```python
from build123d import *

# Parameters (mm, degrees)
DODANIE_WYCI_GNI_CIE1_DEPTH      = 0.5
DODANIE_WYCI_GNI_CIE1_DEPTH_BACK = 2
DODANIE_WYCI_GNI_CIE2_DEPTH      = 5.5
DODANIE_WYCI_GNI_CIE3_DEPTH      = 1.5
ZAOKR_GLENIE1_R                  = 2
SZKIC6_W                         = 66.685530181
SZKIC6_H                         = 2.4
DODANIE_WYCI_GNI_CIE4_DEPTH      = 8.59
DODANIE_WYCI_GNI_CIE5_DEPTH      = 8.59
WYTNIJ_WYCI_GNI_CIE1_DEPTH       = 5.5
SZKIC13_R                        = 3.55
SZKIC13_R_2                      = 1.6
SZKIC13_R_3                      = 1.55
DODANIE_WYCI_GNI_CIE7_DEPTH      = 1.57
SZKIC13_3_R                      = 1.55
WYTNIJ_WYCI_GNI_CIE2_DEPTH       = 90.285917207
WYTNIJ_WYCI_GNI_CIE3_DEPTH       = 2
SFAZOWANIE1_SIZE                 = 1.7


with BuildPart() as part:
    # Szkic3 → Dodanie-wyciągnięcie1 (new, two sides: drawn at the far end of the back side and taken through both)
    with BuildSketch(Plane(origin=(0, 0, -8.74), x_dir=(-1, 0, 0), z_dir=(0, 0, -1)).offset(-DODANIE_WYCI_GNI_CIE1_DEPTH_BACK)):
        Polygon((55.692889856, -69.15246634), (55.692892168, 60.038263946), (-55.811722529, 60.038263946), (-55.811687853, -69.161116694), align=None)
    extrude(amount=DODANIE_WYCI_GNI_CIE1_DEPTH + DODANIE_WYCI_GNI_CIE1_DEPTH_BACK)

    # Szkic4 → Dodanie-wyciągnięcie2 (add)
    with BuildSketch(Plane.XY.offset(-6.74)):
        Polygon((53.802147291, -67.151419689), (53.80218089, 58.038263946), (-53.683348754, 58.038263946), (-53.683348754, -67.143081129), align=None)
        Polygon((51.802147827, -65.151264526), (51.802180354, 56.038263946), (-51.683348754, 56.038263946), (-51.683348754, -65.14323628), align=None, mode=Mode.SUBTRACT)
    extrude(amount=DODANIE_WYCI_GNI_CIE2_DEPTH)

    # Szkic4<3> → Dodanie-wyciągnięcie3 (add)
    with BuildSketch(Plane.XY.offset(-6.74)):
        Polygon((-55.692892168, 60.038263946), (-55.692889856, -69.15246634), (55.811687853, -69.161116694), (55.811722529, 60.038263946), align=None)
        Polygon((-53.683348754, -67.143081129), (-53.683348754, 58.038263946), (53.80218089, 58.038263946), (53.802147291, -67.151419689), align=None, mode=Mode.SUBTRACT)
    extrude(amount=DODANIE_WYCI_GNI_CIE3_DEPTH)

    # Zaokrąglenie1
    zaokr_glenie1_edges = [part.edges().sort_by_distance(p)[0] for p in [
        (53.80218089, 58.038263946, -3.24),
        (-53.683348754, 58.038263946, -3.24),
        (-53.683348754, -67.143081129, -3.24),
        (53.802147291, -67.151419689, -3.24),
        (55.811687853, -69.161116694, -7.24),
        (55.811722529, 60.038263946, -7.24),
        (-55.692892168, 60.038263946, -7.24),
        (-55.692889856, -69.15246634, -7.24),
    ]]
    fillet(zaokr_glenie1_edges, radius=ZAOKR_GLENIE1_R)

    # Szkic6 → Dodanie-wyciągnięcie4 (add)
    with BuildSketch(Plane.XY.offset(-6.74)):
        with Locations((0.159416337, 58.838263946)):
            Rectangle(SZKIC6_W, SZKIC6_H)
    extrude(amount=DODANIE_WYCI_GNI_CIE4_DEPTH)

    # Szkic7 → Dodanie-wyciągnięcie5 (add)
    with BuildSketch(Plane.XY.offset(-6.74)):
        Polygon((-51.683348754, 55.738263946), (51.802180273, 55.738263946), (51.802180354, 56.038263946), (-51.683348754, 56.038263946), align=None)
    extrude(amount=DODANIE_WYCI_GNI_CIE5_DEPTH)

    # Szkic9 → Wytnij-wyciągnięcie1 (cut)
    with BuildSketch(Plane.XZ.offset(-55.738263946)):
        Polygon((51.802180273, 1.85), (38.175466286, 1.85), (44.80199267, -1.24), (51.80199267, -1.24), (51.802180273, -1.24), align=None)
        Polygon((-38.056977527, 1.85), (-51.683348754, 1.85), (-51.683348754, -1.24), (-44.683503911, -1.24), align=None)
    extrude(amount=-WYTNIJ_WYCI_GNI_CIE1_DEPTH, mode=Mode.SUBTRACT)

    # Szkic13 → Dodanie-wyciągnięcie7 (add)
    # profile 1 of 8: a face of its own
    with BuildSketch(Plane.XY.offset(-6.74)):
        with Locations((-47.14, 47.6022)):
            Circle(SZKIC13_R)
        with Locations((-47.14, 47.6022)):
            Circle(SZKIC13_R_2, mode=Mode.SUBTRACT)
    # profile 2 of 8: a face of its own
    with BuildSketch(Plane.XY.offset(-6.74)):
        with Locations((-47.14, 47.6022)):
            Circle(SZKIC13_R_2)
        with Locations((-47.14, 47.6022)):
            Circle(SZKIC13_R_3, mode=Mode.SUBTRACT)
    # profile 3 of 8: a face of its own
    with BuildSketch(Plane.XY.offset(-6.74)):
        with Locations((47.352, 47.6022)):
            Circle(SZKIC13_R)
        with Locations((47.352, 47.6022)):
            Circle(SZKIC13_R_2, mode=Mode.SUBTRACT)
    # profile 4 of 8: a face of its own
    with BuildSketch(Plane.XY.offset(-6.74)):
        with Locations((47.352, 47.6022)):
            Circle(SZKIC13_R_2)
        with Locations((47.352, 47.6022)):
            Circle(SZKIC13_R_3, mode=Mode.SUBTRACT)
    # profile 5 of 8: a face of its own
    with BuildSketch(Plane.XY.offset(-6.74)):
        with Locations((-47.14, -58.1478)):
            Circle(SZKIC13_R)
        with Locations((-47.14, -58.1478)):
            Circle(SZKIC13_R_2, mode=Mode.SUBTRACT)
    # profile 6 of 8: a face of its own
    with BuildSketch(Plane.XY.offset(-6.74)):
        with Locations((-47.14, -58.1478)):
            Circle(SZKIC13_R_2)
        with Locations((-47.14, -58.1478)):
            Circle(SZKIC13_R_3, mode=Mode.SUBTRACT)
    # profile 7 of 8: a face of its own
    with BuildSketch(Plane.XY.offset(-6.74)):
        with Locations((47.352, -58.1478)):
            Circle(SZKIC13_R)
        with Locations((47.352, -58.1478)):
            Circle(SZKIC13_R_2, mode=Mode.SUBTRACT)
    # profile 8 of 8: a face of its own
    with BuildSketch(Plane.XY.offset(-6.74)):
        with Locations((47.352, -58.1478)):
            Circle(SZKIC13_R_2)
        with Locations((47.352, -58.1478)):
            Circle(SZKIC13_R_3, mode=Mode.SUBTRACT)
    extrude(amount=DODANIE_WYCI_GNI_CIE7_DEPTH)

    # Szkic13<3> → Wytnij-wyciągnięcie2 (cut, through all)
    with BuildSketch(Plane.XY.offset(-6.74)):
        with Locations((-47.14, -58.1478)):
            Circle(SZKIC13_3_R)
        with Locations((-47.14, 47.6022)):
            Circle(SZKIC13_3_R)
        with Locations((47.352, 47.6022)):
            Circle(SZKIC13_3_R)
        with Locations((47.352, -58.1478)):
            Circle(SZKIC13_3_R)
    extrude(amount=-WYTNIJ_WYCI_GNI_CIE2_DEPTH, mode=Mode.SUBTRACT)

    # Szkic18 → Wytnij-wyciągnięcie3 (cut)
    with BuildSketch(Plane(origin=(-0.00520918, -67.147245397, 0), x_dir=(0.999999996990791, -7.757846392237927e-05, 0), z_dir=(-7.757846392237927e-05, -0.999999996990791, 0))):
        with BuildLine():
            ThreePointArc((-42.245261471, -1.24), (-41.074504923, -2.078778872), (-39.665102055, -2.375097025))
            Line((-39.665102055, -2.375097025), (-34.665098037, -2.375097025))
            ThreePointArc((-34.665098037, -2.375097025), (-33.255694971, -2.078778946), (-32.084938256, -1.24))
            Line((-32.084938256, -1.24), (-42.245261471, -1.24))
        make_face()
    extrude(amount=-WYTNIJ_WYCI_GNI_CIE3_DEPTH, mode=Mode.SUBTRACT)

    # Sfazowanie1
    sfazowanie1_edges = [part.edges().sort_by_distance(p)[0] for p in [
        (45.802, -58.1478, -9.24),
        (45.802, 47.6022, -9.24),
        (-48.69, 47.6022, -9.24),
        (-48.69, -58.1478, -9.24),
    ]]
    chamfer(sfazowanie1_edges, length=SFAZOWANIE1_SIZE)


solid = part.part
```
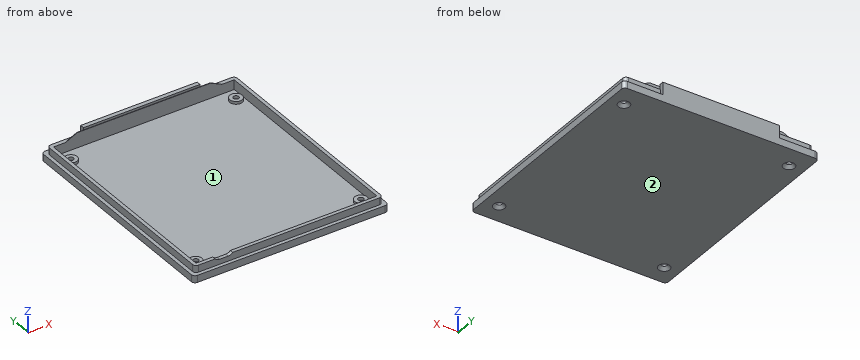
Check sheet for the modelled part. Datum: model origin and axes. Units: mm. Face numbers are marked on the shaded views. Coordinates: 2 decimals unless noted, no trailing zeros. Order: outer loops, then holes, each group sorted by start corner. A loop starts at its lowest first (then second) coordinate and runs counter-clockwise, first axis right, second up. Notation, with made-up numbers: (70.25, 87) -> (80.25, 87) arc R29 ccw to (80.25, 114) -> close; hole circle Ø2 at (54.25, 25). An arc over 180 degrees is marked (long way). Write item = value, one per line. Start each with the question number.
1) Material ranges on L1, parallel to Y at x = -47.14, z = -7.15; L2, parallel to X at y = -12, z = -5; L3, parallel to Y at x = -47.14, z = -6.4, recorded low to high.
2) Go/stop test with flat-tipped pins: P1, Ø2, axis at x = 49, y = -56.5, coming from the +Z side; P2, Ø6, axis at x = 8.5, z = -3.5, coming from the -Y side; P3, Ø3.5, axis at x = 8.5, z = 0, coming from the -Y side. Record where each tip stops, or that it passes through.
3) Mould release check, pull along X, two halves, no side actions. Record for the marked faces 1 and 2: +X half, -X half, draft (parallel to the pull), parting line (faces both ways), or undercut.
4) Cross-section at A-A (x = -47.14). State how many separate pieces and enclosed holes the cut face has, then the cut area to 3 significant figures.
5) Cross-section at C-C (x = 8). Enter the section's corners in (y, z).
6) Cross-section at B-B (y = 16). Enter the section's corners in (x, z), then the cut area to 3 significant figures.
Ans:
q1.L1 = -69.15 to -59.7, -56.6 to 46.05, 49.15 to 60.04
q1.L2 = -53.68 to -51.68, 51.8 to 53.8
q1.L3 = -69.15 to -65.14, -61.7 to -59.7, -56.6 to -54.6, 44.05 to 46.05, 49.15 to 51.15, 55.74 to 60.04
q2.P1 = -5.17
q2.P2 = -69.16
q2.P3 = -67.15
q3.face_1 = undercut
q3.face_2 = draft
q4.separate_pieces = 3
q4.enclosed_holes = 0
q4.area = 344 mm²
q5.outline = (-69.16, -9.24) -> (60.04, -9.24) -> (60.04, 1.85) -> (57.64, 1.85) -> (57.64, -1.24) -> (56.04, -1.24) -> (56.04, 1.85) -> (55.74, 1.85) -> (55.74, -6.74) -> (-65.15, -6.74) -> (-65.15, -1.24) -> (-67.15, -1.24) -> (-67.15, -5.24) -> (-69.16, -5.24) -> close
q6.outline = (-55.69, -9.24) -> (55.81, -9.24) -> (55.81, -5.24) -> (53.8, -5.24) -> (53.8, -1.24) -> (51.8, -1.24) -> (51.8, -6.74) -> (-51.68, -6.74) -> (-51.68, -1.24) -> (-53.68, -1.24) -> (-53.68, -5.24) -> (-55.69, -5.24) -> close
q6.area = 307 mm²
